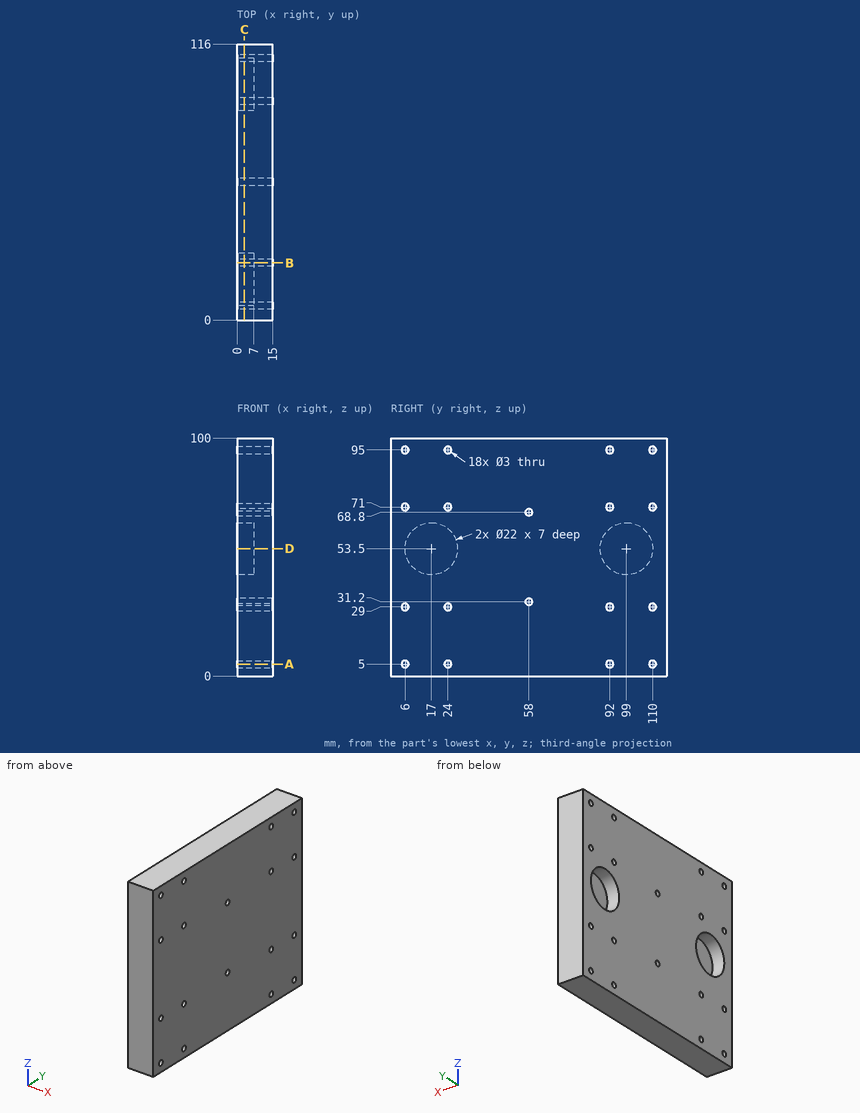
Print and shaded views of the part. All mm, measured from the part's lowest x, y and z. Round coordinates to 2 decimals unless told otherwise and drop trailing zeros. Write each loop counter-clockwise with the first axis right and the second up, starting at its lowest first coordinate (ties: lowest second). Pieces come first, ordered by that corner, then holes. Notation, with made-up numbers: (-20, -1) - (27, -1) arc R30 cw to (27, 30) - close; hole circle Ø4 at (80, 46). An arc over 180 degrees is marked (long way). Write each question's results on one line, items separated by ' | '. Start each with the question number.
Item 1: Saw through at D-D (z = 53.5). Write the cut outline in (x, y), and give its area (3 significant figures).
Item 2: Saw through at A-A (z = 5). Write the cut outline in (x, y).
Item 3: Saw through at B-B (y = 24). Write the cut outline in (x, z), and give its area (3 significant figures).
Item 4: Wall check: L1, parallel to Y at x = 6.75, z = 29; L2, parallel to Z at x = 10.5, y = 110; L3, parallel to Z at x = 1.25, y = 24.5. Give the ranges that are in metal, low to high. Write a range as [from, to].
Item 5: Saw through at C-C (x = 3). State how many separate pieces and enclosed holes the cut face has, and give its area (3 significant figures).
Item 6: Drop flat-ended pins along their axis: P1, Ø1.5, axis at x = 2, y = 80.5, coming from the -Z side; P2, Ø6.5, axis at y = 12, z = 49.5, coming from the -X side. Give the stop position or say it passes through.
Results are:
1) outline: (0, 0) - (15, 0) - (15, 116) - (0, 116) - (0, 110) - (7, 110) - (7, 88) - (0, 88) - (0, 28) - (7, 28) - (7, 6) - (0, 6) - close | area: 1,430 mm²
2) outline: (0, 0) - (15, 0) - (15, 4.5) - (0, 4.5) - close; (0, 7.5) - (15, 7.5) - (15, 22.5) - (0, 22.5) - close; (0, 25.5) - (15, 25.5) - (15, 90.5) - (0, 90.5) - close; (0, 93.5) - (15, 93.5) - (15, 108.5) - (0, 108.5) - close; (0, 111.5) - (15, 111.5) - (15, 116) - (0, 116) - close
3) outline: (0, 0) - (15, 0) - (15, 3.5) - (0, 3.5) - close; (0, 6.5) - (15, 6.5) - (15, 27.5) - (0, 27.5) - close; (0, 30.5) - (15, 30.5) - (15, 69.5) - (0, 69.5) - (0, 61.99) - (7, 61.99) - (7, 45.01) - (0, 45.01) - close; (0, 72.5) - (15, 72.5) - (15, 93.5) - (0, 93.5) - close; (0, 96.5) - (15, 96.5) - (15, 100) - (0, 100) - close | area: 1,200 mm²
4) L1: y = [0, 4.5], [7.5, 22.5], [25.5, 90.5], [93.5, 108.5], [111.5, 116] | L2: z = [0, 3.5], [6.5, 27.5], [30.5, 69.5], [72.5, 93.5], [96.5, 100] | L3: z = [0, 3.59], [6.41, 27.59], [30.41, 45.45], [61.55, 69.59], [72.41, 93.59], [96.41, 100]
5) separate pieces: 1 | enclosed holes: 20 | area: 10,700 mm²
6) P1: stops at z = 0 | P2: stops at x = 7
